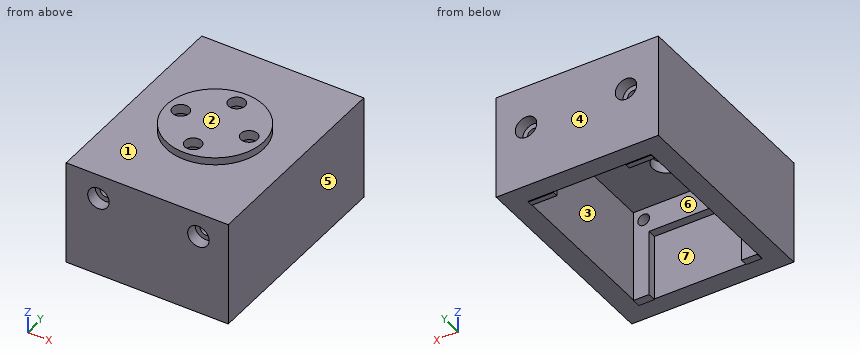
```python
from build123d import *

# Parameters (mm, degrees)
SKETCH1_R                                           = 9.975
BOSS_EXTRUDE1_DEPTH                                 = 1.5
SKETCH3_W                                           = 25.23
SKETCH3_H                                           = 35.5
BOSS_EXTRUDE4_DEPTH                                 = 2.65
SKETCH3_5_W                                         = 33.23
SKETCH3_5_H                                         = 43.5
SKETCH3_5_W_2                                       = 25.23
SKETCH3_5_H_2                                       = 35.5
BOSS_EXTRUDE5_DEPTH                                 = 21.4
SKETCH4_W                                           = 5.2
SKETCH4_H                                           = 1.1
SKETCH4_W_2                                         = 3.2
SKETCH4_H_2                                         = 1.5
SKETCH4_H_3                                         = 1.75
BOSS_EXTRUDE6_DEPTH                                 = 18.9
SKETCH6_W                                           = 18.83
SKETCH6_H                                           = 1.75
BOSS_EXTRUDE7_DEPTH                                 = 5.3
SKETCH2_R                                           = 1.6
CUT_EXTRUDE1_DEPTH                                  = 37
CBORE_FOR_M3_HEX_SOCKET_HEAD_CAP_SCREW1_D           = 3.4
CBORE_FOR_M3_HEX_SOCKET_HEAD_CAP_SCREW1_DEPTH       = 4.15
CBORE_FOR_M3_HEX_SOCKET_HEAD_CAP_SCREW1_CBORE_D     = 5.8
CBORE_FOR_M3_HEX_SOCKET_HEAD_CAP_SCREW1_CBORE_DEPTH = 2.2
CBORE_FOR_M2_HEX_SOCKET_HEAD_CAP_SCREW1_D           = 2.4
CBORE_FOR_M2_HEX_SOCKET_HEAD_CAP_SCREW1_DEPTH       = 6.5
CBORE_FOR_M2_HEX_SOCKET_HEAD_CAP_SCREW1_CBORE_D     = 4.4
CBORE_FOR_M2_HEX_SOCKET_HEAD_CAP_SCREW1_CBORE_DEPTH = 2.4
CBORE_FOR_M2_HEX_SOCKET_HEAD_CAP_SCREW1_TIP         = 0.721032743
CBORE_FOR_M2_HEX_SOCKET_HEAD_CAP_SCREW2_D           = 2.4
CBORE_FOR_M2_HEX_SOCKET_HEAD_CAP_SCREW2_DEPTH       = 6.5
CBORE_FOR_M2_HEX_SOCKET_HEAD_CAP_SCREW2_CBORE_D     = 4.4
CBORE_FOR_M2_HEX_SOCKET_HEAD_CAP_SCREW2_CBORE_DEPTH = 2.4
CBORE_FOR_M2_HEX_SOCKET_HEAD_CAP_SCREW2_TIP         = 0.721032743


with BuildPart() as part:
    # Sketch1 → Boss-Extrude1 (new body)
    with BuildSketch(Plane.XY):
        Circle(SKETCH1_R)
    extrude(amount=BOSS_EXTRUDE1_DEPTH)

    # Sketch3 → Boss-Extrude4 (add)
    with BuildSketch(Plane(origin=(0, 0, 0), x_dir=(-1, 0, 0), z_dir=(0, 0, -1))):
        Rectangle(SKETCH3_W, SKETCH3_H)
    extrude(amount=BOSS_EXTRUDE4_DEPTH)

    # Sketch3<5> → Boss-Extrude5 (add)
    with BuildSketch(Plane(origin=(0, 0, 0), x_dir=(-1, 0, 0), z_dir=(0, 0, -1))):
        Rectangle(SKETCH3_5_W, SKETCH3_5_H)
        Rectangle(SKETCH3_5_W_2, SKETCH3_5_H_2, mode=Mode.SUBTRACT)
    extrude(amount=BOSS_EXTRUDE5_DEPTH)

    # Sketch4 → Boss-Extrude6 (add)
    with BuildSketch(Plane(origin=(0, 0, -2.65), x_dir=(-1, 0, 0), z_dir=(0, 0, -1))):
        with Locations((10.015, 17.2)):
            Rectangle(SKETCH4_W, SKETCH4_H)
        with Locations((-10.015, 17.2)):
            Rectangle(SKETCH4_W, SKETCH4_H)
        with Locations((11.015, -17)):
            Rectangle(SKETCH4_W_2, SKETCH4_H_2)
        with Locations((-11.015, -16.875)):
            Rectangle(SKETCH4_W_2, SKETCH4_H_3)
    extrude(amount=BOSS_EXTRUDE6_DEPTH)

    # Sketch6 → Boss-Extrude7 (add)
    with BuildSketch(Plane(origin=(0, 0, -2.65), x_dir=(-1, 0, 0), z_dir=(0, 0, -1))):
        with Locations((0, -16.875)):
            Rectangle(SKETCH6_W, SKETCH6_H)
    extrude(amount=BOSS_EXTRUDE7_DEPTH)

    # Sketch2 → Cut-Extrude1 (cut)
    with BuildSketch(Plane.XY.offset(1.5)):
        with Locations((7, 0)):
            Circle(SKETCH2_R)
        with Locations((0, -7)):
            Circle(SKETCH2_R)
        with Locations((-7, 0)):
            Circle(SKETCH2_R)
        with Locations((0, 7)):
            Circle(SKETCH2_R)
    extrude(amount=-CUT_EXTRUDE1_DEPTH, mode=Mode.SUBTRACT)

    # CBORE for M3 Hex Socket Head Cap Screw1
    with Locations(Plane(origin=(0, 0, -2.65), x_dir=(-1, 0, 0), z_dir=(0, 0, -1))):
        with Locations((0, 7.000001873), (-7.000001873, 0), (0, -7), (7, 0)):
            CounterBoreHole(CBORE_FOR_M3_HEX_SOCKET_HEAD_CAP_SCREW1_D / 2, CBORE_FOR_M3_HEX_SOCKET_HEAD_CAP_SCREW1_CBORE_D / 2, CBORE_FOR_M3_HEX_SOCKET_HEAD_CAP_SCREW1_CBORE_DEPTH, depth=CBORE_FOR_M3_HEX_SOCKET_HEAD_CAP_SCREW1_DEPTH)

    # CBORE for M2 Hex Socket Head Cap Screw1
    with Locations(Plane.XZ.offset(21.75)):
        with Locations((-10.005, -5.01), (10.495, -5.01)):
            CounterBoreHole(CBORE_FOR_M2_HEX_SOCKET_HEAD_CAP_SCREW1_D / 2, CBORE_FOR_M2_HEX_SOCKET_HEAD_CAP_SCREW1_CBORE_D / 2, CBORE_FOR_M2_HEX_SOCKET_HEAD_CAP_SCREW1_CBORE_DEPTH, depth=CBORE_FOR_M2_HEX_SOCKET_HEAD_CAP_SCREW1_DEPTH)
            with Locations((0, 0, -(CBORE_FOR_M2_HEX_SOCKET_HEAD_CAP_SCREW1_DEPTH + CBORE_FOR_M2_HEX_SOCKET_HEAD_CAP_SCREW1_TIP / 2))):  # 118° drill point
                Cone(0, CBORE_FOR_M2_HEX_SOCKET_HEAD_CAP_SCREW1_D / 2, CBORE_FOR_M2_HEX_SOCKET_HEAD_CAP_SCREW1_TIP, mode=Mode.SUBTRACT)

    # CBORE for M2 Hex Socket Head Cap Screw2
    with Locations(Plane(origin=(0, 21.75, 0), x_dir=(1, 0, 0), z_dir=(0, 1, 0))):
        with Locations((-10.005, 8.76), (10.495, 8.76)):
            CounterBoreHole(CBORE_FOR_M2_HEX_SOCKET_HEAD_CAP_SCREW2_D / 2, CBORE_FOR_M2_HEX_SOCKET_HEAD_CAP_SCREW2_CBORE_D / 2, CBORE_FOR_M2_HEX_SOCKET_HEAD_CAP_SCREW2_CBORE_DEPTH, depth=CBORE_FOR_M2_HEX_SOCKET_HEAD_CAP_SCREW2_DEPTH)
            with Locations((0, 0, -(CBORE_FOR_M2_HEX_SOCKET_HEAD_CAP_SCREW2_DEPTH + CBORE_FOR_M2_HEX_SOCKET_HEAD_CAP_SCREW2_TIP / 2))):  # 118° drill point
                Cone(0, CBORE_FOR_M2_HEX_SOCKET_HEAD_CAP_SCREW2_D / 2, CBORE_FOR_M2_HEX_SOCKET_HEAD_CAP_SCREW2_TIP, mode=Mode.SUBTRACT)


solid = part.part
```
Design review of the part built by this model. Coordinates are the model's own, in mm. Face numbers are marked on the shaded views. A direction names the side the tool comes from. Give positions to 0.01 mm unless a question says otherwise; leave off trailing zeros. Order: outer loops, then holes, each group sorted by start corner. A loop starts at its lowest first (then second) coordinate and runs counter-clockwise, first axis right, second up. Notation, with made-up numbers: (-23.5, 3) - (28.5, 3) arc R22 cw to (28.5, 14) - close; hole circle Ø2 at (10.5, 84.25). An arc over 180 degrees is marked (long way). Use a Markdown table: item, result. Add a question column.
(1) Add section D-D on z = -1.25. Give the boundary of the cut face in (x, y) (3 decimals).
(2) Mouldability with a two-part tool opening along X and no side actions: class the marked faces 4, 5, 6 and 7 as +X half, -X half, draft (parallel to the pull), parting line (faces both ways), or undercut.
(3) Clearance check with flat-ended pins moving along their axes: P1, Ø1.5, axis at x = 9, y = 9, coming from the -Z side; P2, Ø0.9, axis at x = -1, y = -17, coming from the -Z side; P3, Ø3, axis at x = 11, y = 11.5, coming from the +Z side. State where each tip first meets the part, or that it passes through.
(4) Add section B-B on x = 0. Give the number of separate pieces and of enclosed holes in the cut face, then the cut area to 3 significant figures.
(5) Machinability: for the marked faces 1, 2 and 3, which of the approach directions +Z, -Z, +X, -X, +Y, -Y give a long, thin tool a straight path to every point of the face, cutting with its end or side? Answer none if there is none.
(6) Wall thickness on probe 1 along X at (y, z) = (19.9, -8.76) (3 decimals); probe 2 along X at (y, z) = (8, -16) (3 decimals); probe 3 along Y at (x, z) = (-8.5, -15.5): over which ranges is each line inside the solid? List them lowest first. Write a range as [from, to].
(7) Add section A-A on y = 0. Give the boundary of the cut face in (x, z) (3 decimals).
Report:
| question | item | result |
|---|---|---|
| 1 | outline | (-16.615, -21.75) - (16.615, -21.75) - (16.615, 21.75) - (-16.615, 21.75) - close; hole circle Ø5.8 at (-7, 0); hole circle Ø5.8 at (0, -7); hole circle Ø5.8 at (0, 7); hole circle Ø5.8 at (7, 0) |
| 2 | face 4 | draft |
| 2 | face 5 | +X half |
| 2 | face 6 | undercut |
| 2 | face 7 | undercut |
| 3 | P1 | stops at z = -2.65 |
| 3 | P2 | stops at z = -7.95 |
| 3 | P3 | stops at z = 0 |
| 4 | separate pieces | 3 |
| 4 | enclosed holes | 0 |
| 4 | area | 266 mm² |
| 5 | face 1 | +Z |
| 5 | face 2 | +Z, +X, -X, +Y, -Y |
| 5 | face 3 | -Z |
| 6 | probe 1 | x = [-16.615, -12.205], [-7.805, 8.295], [12.695, 16.615] |
| 6 | probe 2 | x = [-16.615, -12.615], [12.615, 16.615] |
| 6 | probe 3 | y = [-21.75, -17.75], [16.65, 21.75] |
| 7 | outline | (-16.615, -21.4) - (-12.615, -21.4) - (-12.615, -2.65) - (-9.9, -2.65) - (-9.9, -0.45) - (-8.7, -0.45) - (-8.7, 1.5) - (-9.975, 1.5) - (-9.975, 0) - (-16.615, 0) - close; (-5.3, -0.45) - (-4.1, -0.45) - (-4.1, -2.65) - (4.1, -2.65) - (4.1, -0.45) - (5.3, -0.45) - (5.3, 1.5) - (-5.3, 1.5) - close; (8.7, -0.45) - (9.9, -0.45) - (9.9, -2.65) - (12.615, -2.65) - (12.615, -21.4) - (16.615, -21.4) - (16.615, 0) - (9.975, 0) - (9.975, 1.5) - (8.7, 1.5) - close |
